Read the model definition and answer for the solid it produces. Units are mm, in the model's axes. Face numbers are marked on the shaded views. A direction names the side the tool comes from. Give positions to 0.01 mm unless a question says otherwise; leave off trailing zeros. Write each loop counter-clockwise with the first axis right and the second up, starting at its lowest first coordinate (ties: lowest second). Pieces come first, ordered by that corner, then holes. Notation, with made-up numbers: (68.5, 61.25) -> (74.5, 61.25) arc R22 cw to (74.5, 85.25) -> close; hole circle Ø4 at (-3.5, 41.5). An arc over 180 degrees is marked (long way). Put each result on its own line as item: value. Start each with the question number.
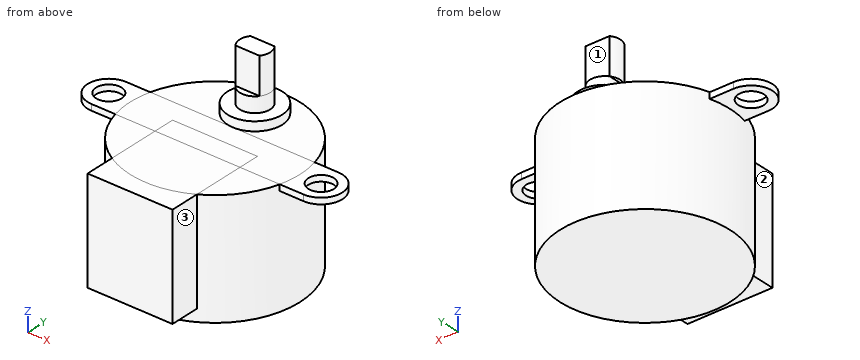
from build123d import *
from build123d.topology import SkipClean

# Parameters (mm, degrees)
SKETCH2_R           = 14
BOSS_EXTRUDE1_DEPTH = 19
SKETCH3_R           = 2.5
BOSS_EXTRUDE2_DEPTH = 4
SKETCH3_3_R         = 4.5
BOSS_EXTRUDE3_DEPTH = 1.5
BOSS_EXTRUDE4_DEPTH = 6
SKETCH6_W           = 14
SKETCH6_H           = 17
BOSS_EXTRUDE5_DEPTH = 17
SKETCH7_R           = 2.1
BOSS_EXTRUDE6_DEPTH = 1


with BuildPart() as part:
    # Sketch2 → Boss-Extrude1 (new body)
    with BuildSketch(Plane.XY):
        Circle(SKETCH2_R)
    extrude(amount=BOSS_EXTRUDE1_DEPTH)

    # Sketch3 → Boss-Extrude2 (add)
    with BuildSketch(Plane.XY.offset(19)):
        with Locations((0, 8)):
            Circle(SKETCH3_R)
    extrude(amount=BOSS_EXTRUDE2_DEPTH)

    # Sketch3<3> → Boss-Extrude3 (add)
    with BuildSketch(Plane.XY.offset(19)):
        with Locations((0, 8)):
            Circle(SKETCH3_3_R)
    extrude(amount=BOSS_EXTRUDE3_DEPTH)

    # Sketch4 → Boss-Extrude4 (add)
    with SkipClean():  # the faces are left unmerged after this step: merging them gives an invalid solid
        with BuildSketch(Plane.XY.offset(23)):
            with BuildLine():
                Line((-2, 9.5), (2, 9.5))
                ThreePointArc((2, 9.5), (2.5, 8), (2, 6.5))
                Line((2, 6.5), (-2, 6.5))
                ThreePointArc((-2, 6.5), (-2.5, 8), (-2, 9.5))
            make_face()
        extrude(amount=BOSS_EXTRUDE4_DEPTH)

    # Sketch6 → Boss-Extrude5 (add)
    with SkipClean():  # the faces are left unmerged after this step: merging them gives an invalid solid
        with BuildSketch(Plane.XY.offset(19)):
            with Locations((0, -8.5)):
                Rectangle(SKETCH6_W, SKETCH6_H)
        extrude(amount=-BOSS_EXTRUDE5_DEPTH)

    # Sketch7 → Boss-Extrude6 (add)
    with SkipClean():  # the faces are left unmerged after this step: merging them gives an invalid solid
        with BuildSketch(Plane.XY.offset(19)):
            with BuildLine():
                Line((-17.5, 3.5), (17.5, 3.5))
                ThreePointArc((17.5, 3.5), (21, 0), (17.5, -3.5))
                Line((17.5, -3.5), (-17.5, -3.5))
                ThreePointArc((-17.5, -3.5), (-21, 0), (-17.5, 3.5))
            make_face()
            with Locations((-17.5, 0)):
                Circle(SKETCH7_R, mode=Mode.SUBTRACT)
            with Locations((17.5, 0)):
                Circle(SKETCH7_R, mode=Mode.SUBTRACT)
        extrude(amount=-BOSS_EXTRUDE6_DEPTH)


solid = part.part
1) Each of these flat-tipped pins is pushed along its axis until it touches: pin 1 Ø3.5 at (x, y) = (-15.5, 1) entering from +Z; pin 2 Ø1.2 at (x, z) = (-0.5, 26) entering from +Y; pin 3 Ø1.5 at (y, z) = (-14.5, 12.5) entering from -X; pin 4 Ø1.5 at (x, y) = (-14.5, -7.5) entering from +Z. Where does it stop, or does it pass through?
2) For the marked faces 1, 2 and 3, determine the directions among +Z, -Z, +X, -X, +Y, -Y from which every point of the face is accessible in a straight line to the end or side of a thin tool.
3) A cutting plane is placed at C-C on z = 26. Give the vertices of the cut face in (x, y), and give its area (3 significant figures).
4) A cutting plane is placed at A-A on y = 1.5. Give the vertices of the cut face in (x, z).
5) A cutting plane is placed at B-B on x = 0. Give the vertices of the cut face in (y, z).
6) Straight lines are drawn through the part: line 1 (Y direction, x = -17.5, z = 18.8); line 2 (Z direction, x = -5.5, y = -12); line 3 (X direction, y = -13.5, z = 15). For each, find the intervals that lie inside material, in ascending order. Write a range as [from, to].
7) A cutting plane is placed at D-D on y = 11. Give the vertices of the cut face in (x, z), and give its area (3 significant figures).
Results found:
1. pin 1: stops at z = 19
1. pin 2: stops at y = 9.5
1. pin 3: stops at x = -7
1. pin 4: passes through
2. face 1: +Z, +X, -X, +Y
2. face 2: +Z, -Z, -X, -Y
2. face 3: +Z, -Z, +X, -Y
3. outline: (-2, 6.5) -> (2, 6.5) arc R2.5 ccw to (2, 9.5) -> (-2, 9.5) arc R2.5 ccw to start
3. area: 14.0 mm²
4. outline: (-20.66, 18) -> (-18.97, 18) -> (-18.97, 19) -> (-20.66, 19) -> close; (-16.03, 18) -> (-13.92, 18) -> (-13.92, 0) -> (13.92, 0) -> (13.92, 18) -> (16.03, 18) -> (16.03, 19) -> (-16.03, 19) -> close; (18.97, 18) -> (20.66, 18) -> (20.66, 19) -> (18.97, 19) -> close
5. outline: (-17, 2) -> (-14, 2) -> (-14, 0) -> (14, 0) -> (14, 19) -> (12.5, 19) -> (12.5, 20.5) -> (10.5, 20.5) -> (10.5, 23) -> (9.5, 23) -> (9.5, 29) -> (6.5, 29) -> (6.5, 23) -> (5.5, 23) -> (5.5, 20.5) -> (3.5, 20.5) -> (3.5, 19) -> (-17, 19) -> close
6. line 1: y = [-3.5, -2.1], [2.1, 3.5]
6. line 2: z = [0, 19]
6. line 3: x = [-7, 7]
7. outline: (-8.66, 0) -> (8.66, 0) -> (8.66, 19) -> (3.35, 19) -> (3.35, 20.5) -> (-3.35, 20.5) -> (-3.35, 19) -> (-8.66, 19) -> close
7. area: 339 mm²
